Read the model definition and answer for the solid it produces. Units are mm, in the model's axes. Round coordinates to 2 decimals unless told otherwise and drop trailing zeros. Order: outer loops, then holes, each group sorted by start corner. A loop starts at its lowest first (then second) coordinate and runs counter-clockwise, first axis right, second up. Notation, with made-up numbers: M 4,84.25 L 49,84.25 A31 cw 49,115.25 Z; hole C 60.5,-13.5 d6. An arc over 180 degrees is marked long. Use one line per item in the form item = value. Start each with the question number.
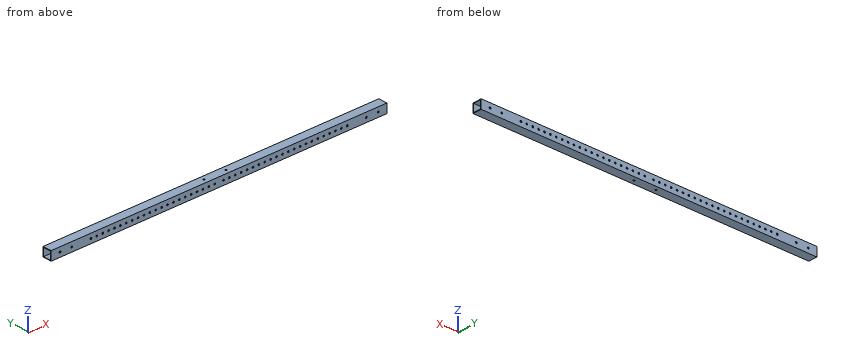
from build123d import *

# Parameters (mm, degrees)
SKETCH_11_W         = 15
SKETCH_11_H         = 15
SKETCH_11_W_2       = 13
SKETCH_11_H_2       = 13
F_15X15X1_1_DEPTH   = 570
SKETCH_12_R         = 1.45
CUT_EXTRUDE_1_DEPTH = 286.49299466
SKETCH_13_R         = 1.45
CUT_EXTRUDE_2_DEPTH = 286.49299466
SKETCH_14_R         = 1.45
CUT_EXTRUDE_3_DEPTH = 286.49299466


with BuildPart() as part:
    # 草图11 → 铝管 15X15X1(1) (new body)
    with BuildSketch(Plane(origin=(-285, 0, 0), x_dir=(0, 0, -1), z_dir=(1, 0, 0))):
        Rectangle(SKETCH_11_W, SKETCH_11_H)
        Rectangle(SKETCH_11_W_2, SKETCH_11_H_2, mode=Mode.SUBTRACT)
    extrude(amount=F_15X15X1_1_DEPTH)

    # 草图12 → 切除-拉伸1 (cut, through all)
    with BuildSketch(Plane(origin=(0, 7.5, 0), x_dir=(1, 0, 0), z_dir=(0, 1, 0))):
        with Locations(Location((-270, 0, 0), (0, 0, 270))):
            Circle(SKETCH_12_R)
        with Locations(Location((-250, 0, 0), (0, 0, 270))):
            Circle(SKETCH_12_R)
        with Locations(Location((250, 0, 0), (0, 0, 90))):
            Circle(SKETCH_12_R)
        with Locations(Location((270, 0, 0), (0, 0, 90))):
            Circle(SKETCH_12_R)
    extrude(amount=-CUT_EXTRUDE_1_DEPTH, mode=Mode.SUBTRACT)

    # 草图13 → 切除-拉伸2 (cut, through all)
    with BuildSketch(Plane(origin=(0, 0, -7.5), x_dir=(-1, 0, 0), z_dir=(0, 0, -1))):
        with Locations((-18.5, 0)):
            Circle(SKETCH_13_R)
        with Locations((18.5, 0)):
            Circle(SKETCH_13_R)
    extrude(amount=-CUT_EXTRUDE_2_DEPTH, mode=Mode.SUBTRACT)

    # 草图14 → 切除-拉伸3 (cut, through all)
    with BuildSketch(Plane.XZ.offset(7.5)):
        with Locations(Location((-97.5, 0, 0), (0, 0, 270))):
            Circle(SKETCH_14_R)
        with Locations(Location((-87.5, 0, 0), (0, 0, 270))):
            Circle(SKETCH_14_R)
        with Locations(Location((-117.5, 0, 0), (0, 0, 270))):
            Circle(SKETCH_14_R)
        with Locations(Location((-107.5, 0, 0), (0, 0, 270))):
            Circle(SKETCH_14_R)
        with Locations(Location((-137.5, 0, 0), (0, 0, 270))):
            Circle(SKETCH_14_R)
        with Locations(Location((-127.5, 0, 0), (0, 0, 270))):
            Circle(SKETCH_14_R)
        with Locations(Location((-157.5, 0, 0), (0, 0, 270))):
            Circle(SKETCH_14_R)
        with Locations(Location((-147.5, 0, 0), (0, 0, 270))):
            Circle(SKETCH_14_R)
        with Locations(Location((-177.5, 0, 0), (0, 0, 270))):
            Circle(SKETCH_14_R)
        with Locations(Location((-167.5, 0, 0), (0, 0, 270))):
            Circle(SKETCH_14_R)
        with Locations(Location((-197.5, 0, 0), (0, 0, 270))):
            Circle(SKETCH_14_R)
        with Locations(Location((-187.5, 0, 0), (0, 0, 270))):
            Circle(SKETCH_14_R)
        with Locations(Location((-217.5, 0, 0), (0, 0, 270))):
            Circle(SKETCH_14_R)
        with Locations(Location((-207.5, 0, 0), (0, 0, 270))):
            Circle(SKETCH_14_R)
        with Locations(Location((-77.5, 0, 0), (0, 0, 270))):
            Circle(SKETCH_14_R)
        with Locations(Location((-67.5, 0, 0), (0, 0, 270))):
            Circle(SKETCH_14_R)
        with Locations(Location((-57.5, 0, 0), (0, 0, 270))):
            Circle(SKETCH_14_R)
        with Locations(Location((-47.5, 0, 0), (0, 0, 270))):
            Circle(SKETCH_14_R)
        with Locations(Location((-37.5, 0, 0), (0, 0, 270))):
            Circle(SKETCH_14_R)
        with Locations(Location((-27.5, 0, 0), (0, 0, 270))):
            Circle(SKETCH_14_R)
        with Locations(Location((-17.5, 0, 0), (0, 0, 270))):
            Circle(SKETCH_14_R)
        with Locations(Location((-7.5, 0, 0), (0, 0, 270))):
            Circle(SKETCH_14_R)
        with Locations(Location((7.5, 0, 0), (0, 0, 270))):
            Circle(SKETCH_14_R)
        with Locations(Location((17.5, 0, 0), (0, 0, 270))):
            Circle(SKETCH_14_R)
        with Locations(Location((27.5, 0, 0), (0, 0, 270))):
            Circle(SKETCH_14_R)
        with Locations(Location((37.5, 0, 0), (0, 0, 270))):
            Circle(SKETCH_14_R)
        with Locations(Location((47.5, 0, 0), (0, 0, 270))):
            Circle(SKETCH_14_R)
        with Locations(Location((57.5, 0, 0), (0, 0, 270))):
            Circle(SKETCH_14_R)
        with Locations(Location((67.5, 0, 0), (0, 0, 270))):
            Circle(SKETCH_14_R)
        with Locations(Location((77.5, 0, 0), (0, 0, 270))):
            Circle(SKETCH_14_R)
        with Locations(Location((207.5, 0, 0), (0, 0, 270))):
            Circle(SKETCH_14_R)
        with Locations(Location((217.5, 0, 0), (0, 0, 270))):
            Circle(SKETCH_14_R)
        with Locations(Location((187.5, 0, 0), (0, 0, 270))):
            Circle(SKETCH_14_R)
        with Locations(Location((197.5, 0, 0), (0, 0, 270))):
            Circle(SKETCH_14_R)
        with Locations(Location((167.5, 0, 0), (0, 0, 270))):
            Circle(SKETCH_14_R)
        with Locations(Location((177.5, 0, 0), (0, 0, 270))):
            Circle(SKETCH_14_R)
        with Locations(Location((147.5, 0, 0), (0, 0, 270))):
            Circle(SKETCH_14_R)
        with Locations(Location((157.5, 0, 0), (0, 0, 270))):
            Circle(SKETCH_14_R)
        with Locations(Location((127.5, 0, 0), (0, 0, 270))):
            Circle(SKETCH_14_R)
        with Locations(Location((137.5, 0, 0), (0, 0, 270))):
            Circle(SKETCH_14_R)
        with Locations(Location((107.5, 0, 0), (0, 0, 270))):
            Circle(SKETCH_14_R)
        with Locations(Location((117.5, 0, 0), (0, 0, 270))):
            Circle(SKETCH_14_R)
        with Locations(Location((87.5, 0, 0), (0, 0, 270))):
            Circle(SKETCH_14_R)
        with Locations(Location((97.5, 0, 0), (0, 0, 270))):
            Circle(SKETCH_14_R)
    extrude(amount=-CUT_EXTRUDE_3_DEPTH, mode=Mode.SUBTRACT)


solid = part.part
Item 1: Find the intervals of material crossed by L1, parallel to Z at x = -122.5, y = -0.75; L2, parallel to Z at x = -147.5, y = 7, in increasing order. Write a range as [from, to].
Item 2: Given P1, Ø2.5, axis at x = 167.5, z = 0, coming from the +Y side, flat-ended and moving along its own axis, determine where the tip first touches the part or whether it passes through.
Item 3: Section A-A (y = -4.25) is taken. Write down the section's boundary in (x, z).
Item 4: Section B-B (x = 241.5) is taken. Write down the section's boundary in (y, z), and give its area (3 significant figures).
The answers:
q1.L1 = [-7.5, -6.5], [6.5, 7.5]
q1.L2 = [-7.5, -1.45], [1.45, 7.5]
q2.P1 = through
q3.outline = M -285,-7.5 L 285,-7.5 L 285,-6.5 L -285,-6.5 Z; M -285,6.5 L 285,6.5 L 285,7.5 L -285,7.5 Z
q4.outline = M -7.5,-7.5 L 7.5,-7.5 L 7.5,7.5 L -7.5,7.5 Z; hole M -6.5,-6.5 L 6.5,-6.5 L 6.5,6.5 L -6.5,6.5 Z
q4.area = 56.0 mm²
